Part model, mm, in its own coordinate system. A direction names the side the tool comes from. Round coordinates to 2 decimals unless told otherwise and drop trailing zeros. Write each loop counter-clockwise with the first axis right and the second up, starting at its lowest first coordinate (ties: lowest second). Pieces come first, ordered by that corner, then holes. Notation, with made-up numbers: (-10.75, 3.5) -> (27.25, 3.5) arc R32 ccw to (27.25, 34.5) -> close; hole circle Ø8 at (-18.75, -32). An arc over 180 degrees is marked (long way). Return JSON: item names as keys, results as strings. Group by question number.
(1) Tool access for faces 1 (the flat face through (112.395, 0, 41)), 2 (the flat face through (-123.825, 0, -32)), 3 (the flat face through (-149.225, 0, -40)): list every direction of +Z, -Z, +X, -X, +Y, -Y with a clear straight run to the whole face (end or side of a thin tool).
(2) Drop flat-ended pins along their axis: pin 1 Ø3 at (y, z) = (1, -36.5) entering from +X (3 decimals); pin 2 Ø1 at (y, z) = (-0.5, -4) entering from +X (3 decimals); pin 3 Ø3 at (y, z) = (0.5, -0.5) entering from -X (3 decimals). Give the stop position or say it passes through.
(3) Saw through at D-D (x = -106). List the corners of the cut face in (y, z) (3 decimals), plus the area to 3 significant figures.
(4) Saw through at C-C (y = 1.25). State how many separate pieces and enclosed holes the cut face has, plus the area to 3 significant figures.
(5) Saw through at A-A (x = 115). List the corners of the cut face in (y, z) (3 decimals).
(6) Saw through at B-B (z = 4.5). List the corners of the cut face in (x, y) (3 decimals), plus the area to 3 significant figures.
(7) Drill centre lines: L1, parallel to X at y = -0.75, z = -11.5 (3 decimals); L2, parallel to X at y = 1, z = -34.5 (3 decimals); L3, parallel to Z at x = -137, y = 2.5. Where is each one in solid material? Low to high. Write a range as from..to.
from build123d import *

# Parameters (mm, degrees)
BOSS_EXTRUDE1_DEPTH     = 3.175
SKETCH2_W               = 6.35
SKETCH2_H               = 25.4
CUT_EXTRUDE1_DEPTH      = 4.175
CUT_EXTRUDE1_DEPTH_BACK = 4.175


with BuildPart() as part:
    # Sketch1 → Boss-Extrude1 (new body, symmetric)
    with BuildSketch(Plane(origin=(0, 0, 0), x_dir=(1, 0, 0), z_dir=(0, 1, 0))):
        Polygon((149.225, -44.45), (112.395, -44.45), (112.395, -38.1), (97.155, -38.1), (97.155, -44.45), (-149.225, -44.45), (-149.225, -34.874677354), (-152.4, -34.874677354), (-152.4, -14.046677354), (-149.225, -14.046677354), (-149.225, -10.414), (-128.905, -10.414), (-128.905, 10.414), (-149.225, 10.414), (-149.225, 14.046677354), (-152.4, 14.046677354), (-152.4, 34.874677354), (-149.225, 34.874677354), (-149.225, 44.45), (-123.825, 44.45), (-123.825, 19.05), (-98.425, 19.05), (-98.425, 44.45), (98.425, 44.45), (98.425, 19.05), (123.825, 19.05), (123.825, 44.45), (149.225, 44.45), (149.225, 34.874677354), (152.4, 34.874677354), (152.4, 14.046677354), (149.225, 14.046677354), (149.225, 10.414), (128.905, 10.414), (128.905, -10.414), (149.225, -10.414), (149.225, -14.046677354), (152.4, -14.046677354), (152.4, -34.874677354), (149.225, -34.874677354), align=None)
    extrude(amount=BOSS_EXTRUDE1_DEPTH, both=True)

    # Sketch2 → Cut-Extrude1 (cut, two sides)
    with BuildSketch(Plane(origin=(0, 0, 0), x_dir=(1, 0, 0), z_dir=(0, 1, 0))) as cut_extrude1_sk:
        with Locations((115.57, 0)):
            Rectangle(SKETCH2_W, SKETCH2_H)
        with Locations((-115.57, 0)):
            Rectangle(SKETCH2_W, SKETCH2_H)
    extrude(amount=CUT_EXTRUDE1_DEPTH, mode=Mode.SUBTRACT)
    extrude(cut_extrude1_sk.sketch, amount=-CUT_EXTRUDE1_DEPTH_BACK, mode=Mode.SUBTRACT)


solid = part.part
Computed values:
{
 "1": {"face 1": "+Z, +Y, -Y", "face 2": "-Z, +Y, -Y", "face 3": "-Z, -X, +Y, -Y"},
 "2": {"pin 1": "x = 149.225", "pin 2": "x = 128.905", "pin 3": "x = -128.905"},
 "3": {"outline": "(-3.175, -19.05) -> (3.175, -19.05) -> (3.175, 44.45) -> (-3.175, 44.45) -> close", "area": "403 mm2"},
 "4": {"separate pieces": "1", "enclosed holes": "2", "area": "24,200 mm2"},
 "5": {"outline": "(-3.175, -19.05) -> (3.175, -19.05) -> (3.175, -12.7) -> (-3.175, -12.7) -> close; (-3.175, 12.7) -> (3.175, 12.7) -> (3.175, 44.45) -> (-3.175, 44.45) -> close"},
 "6": {"outline": "(-128.905, -3.175) -> (-118.745, -3.175) -> (-118.745, 3.175) -> (-128.905, 3.175) -> close; (-112.395, -3.175) -> (112.395, -3.175) -> (112.395, 3.175) -> (-112.395, 3.175) -> close; (118.745, -3.175) -> (128.905, -3.175) -> (128.905, 3.175) -> (118.745, 3.175) -> close", "area": "1,560 mm2"},
 "7": {"L1": "-149.225..-118.745, -112.395..112.395, 118.745..149.225", "L2": "-152.4..-123.825, -98.425..98.425, 123.825..152.4", "L3": "-44.45..-10.41, 10.41..44.45"}
}
